```python
from build123d import *

# Parameters (mm, degrees)
F0_W         = 38.1
F0_H         = 38.1
F1_DEPTH     = 869.95
F2_W         = 12.7
F2_H         = 114.3
F2_H_2       = 25.4
F3_DEPTH     = 14.2875
F4_W         = 12.7
F4_H         = 114.3
F4_H_2       = 25.4
F5_DEPTH     = 14.2875
F6_T1_DEPTH  = 30.1625
F6_T3_DEPTH  = 12.7
F6_T5_DEPTH  = 30.1625
F6_T7_DEPTH  = 12.7
F6_T13_DEPTH = 28.575
F6_T17_DEPTH = 28.575
F6_T24_DEPTH = 28.575
F6_T28_DEPTH = 28.575
F6_T35_DEPTH = 28.575
F6_T39_DEPTH = 28.575
F6_T46_DEPTH = 28.575
F6_T50_DEPTH = 28.575


# Not quite as in the source:
# - a fillet or chamfer that OpenCascade refuses, or shapes differently, is made with other operations: its cross-section is extruded or revolved along the edge and cut away or added


with BuildPart() as f1:
    # F0 (on Top) → F1 (new body)
    with BuildSketch(Plane.XY):
        Rectangle(F0_W, F0_H)
    extrude(amount=-F1_DEPTH)

    # F2 (on face) → F3 (cut)
    with BuildSketch(Plane.XZ.offset(19.05)):
        with Locations((0, -76.2)):
            Rectangle(F2_W, F2_H)
        with Locations((0, -609.6)):
            Rectangle(F2_W, F2_H_2)
    extrude(amount=-F3_DEPTH, mode=Mode.SUBTRACT)

    # F4 (on face) → F5 (cut)
    with BuildSketch(Plane.YZ.offset(19.05)):
        with Locations((0, -76.2)):
            Rectangle(F4_W, F4_H)
        with Locations((0, -609.6)):
            Rectangle(F4_W, F4_H_2)
    extrude(amount=-F5_DEPTH, mode=Mode.SUBTRACT)

    # F6: fillet of radius 6.35 on 16 edges, made by hand

    # F6_s2 → F6_t1 (join)
    with BuildSketch(Plane.XZ.offset(-11.1125)):
        with BuildLine():
            ThreePointArc((-6.35, -25.4), (-4.4901280605, -20.9098719395), (0, -19.05))
            Line((0, -19.05), (-6.35, -19.05))
            Line((-6.35, -19.05), (-6.35, -25.4))
        make_face()
        with BuildLine():
            ThreePointArc((-6.35, -127), (-4.4901280605, -131.4901280605), (0, -133.35))
            Line((0, -133.35), (-6.35, -133.35))
            Line((-6.35, -133.35), (-6.35, -127))
        make_face()
        with BuildLine():
            ThreePointArc((-6.35, -603.25), (-4.4901280605, -598.7598719395), (0, -596.9))
            Line((0, -596.9), (-6.35, -596.9))
            Line((-6.35, -596.9), (-6.35, -603.25))
        make_face()
        with BuildLine():
            ThreePointArc((-6.35, -615.95), (-4.4901280605, -620.4401280605), (0, -622.3))
            Line((0, -622.3), (-6.35, -622.3))
            Line((-6.35, -622.3), (-6.35, -615.95))
        make_face()
    extrude(amount=F6_T1_DEPTH)

    # F6_s4 → F6_t3 (join)
    with BuildSketch(Plane.XZ.offset(6.35)):
        with BuildLine():
            ThreePointArc((6.35, -25.4), (4.4901280605, -20.9098719395), (0, -19.05))
            Line((0, -19.05), (6.35, -19.05))
            Line((6.35, -19.05), (6.35, -25.4))
        make_face()
        with BuildLine():
            ThreePointArc((0, -133.35), (4.4901280605, -131.4901280605), (6.35, -127))
            Line((6.35, -127), (6.35, -133.35))
            Line((6.35, -133.35), (0, -133.35))
        make_face()
        with BuildLine():
            ThreePointArc((6.35, -603.25), (4.4901280605, -598.7598719395), (0, -596.9))
            Line((0, -596.9), (6.35, -596.9))
            Line((6.35, -596.9), (6.35, -603.25))
        make_face()
        with BuildLine():
            ThreePointArc((0, -622.3), (4.4901280605, -620.4401280605), (6.35, -615.95))
            Line((6.35, -615.95), (6.35, -622.3))
            Line((6.35, -622.3), (0, -622.3))
        make_face()
    extrude(amount=F6_T3_DEPTH)

    # F6_s6 → F6_t5 (join)
    with BuildSketch(Plane.YZ.offset(-11.1125)):
        with BuildLine():
            ThreePointArc((0, -133.35), (4.4901280605, -131.4901280605), (6.35, -127))
            Line((6.35, -127), (6.35, -133.35))
            Line((6.35, -133.35), (0, -133.35))
        make_face()
        with BuildLine():
            ThreePointArc((0, -19.05), (4.4901280605, -20.9098719395), (6.35, -25.4))
            Line((6.35, -25.4), (6.35, -19.05))
            Line((6.35, -19.05), (0, -19.05))
        make_face()
        with BuildLine():
            ThreePointArc((0, -596.9), (4.4901280605, -598.7598719395), (6.35, -603.25))
            Line((6.35, -603.25), (6.35, -596.9))
            Line((6.35, -596.9), (0, -596.9))
        make_face()
        with BuildLine():
            ThreePointArc((0, -622.3), (4.4901280605, -620.4401280605), (6.35, -615.95))
            Line((6.35, -615.95), (6.35, -622.3))
            Line((6.35, -622.3), (0, -622.3))
        make_face()
    extrude(amount=F6_T5_DEPTH)

    # F6_s8 → F6_t7 (join)
    with BuildSketch(Plane.YZ.offset(6.35)):
        with BuildLine():
            ThreePointArc((0, -133.35), (-4.4901280605, -131.4901280605), (-6.35, -127))
            Line((-6.35, -127), (-6.35, -133.35))
            Line((-6.35, -133.35), (0, -133.35))
        make_face()
        with BuildLine():
            ThreePointArc((0, -19.05), (-4.4901280605, -20.9098719395), (-6.35, -25.4))
            Line((-6.35, -25.4), (-6.35, -19.05))
            Line((-6.35, -19.05), (0, -19.05))
        make_face()
        with BuildLine():
            ThreePointArc((0, -596.9), (-4.4901280605, -598.7598719395), (-6.35, -603.25))
            Line((-6.35, -603.25), (-6.35, -596.9))
            Line((-6.35, -596.9), (0, -596.9))
        make_face()
        with BuildLine():
            ThreePointArc((0, -622.3), (-4.4901280605, -620.4401280605), (-6.35, -615.95))
            Line((-6.35, -615.95), (-6.35, -622.3))
            Line((-6.35, -622.3), (0, -622.3))
        make_face()
    extrude(amount=F6_T7_DEPTH)


with BuildPart() as f6_tool11:
    # F6_s12 → F6_t13 (new body)
    with BuildSketch(Plane.XZ.offset(19.05)):
        with BuildLine():
            ThreePointArc((6.35, -25.4), (4.4901280605, -20.9098719395), (0, -19.05))
            Line((0, -19.05), (6.35, -19.05))
            Line((6.35, -19.05), (6.35, -25.4))
        make_face()
    extrude(amount=-F6_T13_DEPTH)

    split(bisect_by=Plane.XZ.offset(6.35), keep=Keep.BOTTOM)


with BuildPart() as f6_tool15:
    # F6_s16 → F6_t17 (new body)
    with BuildSketch(Plane.YZ.offset(19.05)):
        with BuildLine():
            ThreePointArc((0, -19.05), (-4.4901280605, -20.9098719395), (-6.35, -25.4))
            Line((-6.35, -25.4), (-6.35, -19.05))
            Line((-6.35, -19.05), (0, -19.05))
        make_face()
    extrude(amount=-F6_T17_DEPTH)

    split(bisect_by=Plane.YZ.offset(6.35), keep=Keep.BOTTOM)


with BuildPart() as f6_tool11_1:
    add(f6_tool11.part)

    # F6_t19: intersect F6_tool15
    add(f6_tool15.part, mode=Mode.INTERSECT)


with BuildPart() as f1_1:
    add(f1.part)

    # F6_t9: union F6_tool11
    add(f6_tool11_1.part)


with BuildPart() as f6_tool22:
    # F6_s23 → F6_t24 (new body)
    with BuildSketch(Plane.YZ.offset(19.05)):
        with BuildLine():
            ThreePointArc((0, -133.35), (-4.4901280605, -131.4901280605), (-6.35, -127))
            Line((-6.35, -127), (-6.35, -133.35))
            Line((-6.35, -133.35), (0, -133.35))
        make_face()
    extrude(amount=-F6_T24_DEPTH)

    split(bisect_by=Plane.YZ.offset(6.35), keep=Keep.BOTTOM)


with BuildPart() as f6_tool26:
    # F6_s27 → F6_t28 (new body)
    with BuildSketch(Plane.XZ.offset(19.05)):
        with BuildLine():
            ThreePointArc((0, -133.35), (4.4901280605, -131.4901280605), (6.35, -127))
            Line((6.35, -127), (6.35, -133.35))
            Line((6.35, -133.35), (0, -133.35))
        make_face()
    extrude(amount=-F6_T28_DEPTH)

    split(bisect_by=Plane.XZ.offset(6.35), keep=Keep.BOTTOM)


with BuildPart() as f6_tool22_1:
    add(f6_tool22.part)

    # F6_t30: intersect F6_tool26
    add(f6_tool26.part, mode=Mode.INTERSECT)


with BuildPart() as f1_2:
    add(f1_1.part)

    # F6_t20: union F6_tool22
    add(f6_tool22_1.part)


with BuildPart() as f6_tool33:
    # F6_s34 → F6_t35 (new body)
    with BuildSketch(Plane.XZ.offset(19.05)):
        with BuildLine():
            ThreePointArc((6.35, -603.25), (4.4901280605, -598.7598719395), (0, -596.9))
            Line((0, -596.9), (6.35, -596.9))
            Line((6.35, -596.9), (6.35, -603.25))
        make_face()
    extrude(amount=-F6_T35_DEPTH)

    split(bisect_by=Plane.XZ.offset(6.35), keep=Keep.BOTTOM)


with BuildPart() as f6_tool37:
    # F6_s38 → F6_t39 (new body)
    with BuildSketch(Plane.YZ.offset(19.05)):
        with BuildLine():
            ThreePointArc((0, -596.9), (-4.4901280605, -598.7598719395), (-6.35, -603.25))
            Line((-6.35, -603.25), (-6.35, -596.9))
            Line((-6.35, -596.9), (0, -596.9))
        make_face()
    extrude(amount=-F6_T39_DEPTH)

    split(bisect_by=Plane.YZ.offset(6.35), keep=Keep.BOTTOM)


with BuildPart() as f6_tool33_1:
    add(f6_tool33.part)

    # F6_t41: intersect F6_tool37
    add(f6_tool37.part, mode=Mode.INTERSECT)


with BuildPart() as f1_3:
    add(f1_2.part)

    # F6_t31: union F6_tool33
    add(f6_tool33_1.part)


with BuildPart() as f6_tool44:
    # F6_s45 → F6_t46 (new body)
    with BuildSketch(Plane.YZ.offset(19.05)):
        with BuildLine():
            ThreePointArc((0, -622.3), (-4.4901280605, -620.4401280605), (-6.35, -615.95))
            Line((-6.35, -615.95), (-6.35, -622.3))
            Line((-6.35, -622.3), (0, -622.3))
        make_face()
    extrude(amount=-F6_T46_DEPTH)

    split(bisect_by=Plane.YZ.offset(6.35), keep=Keep.BOTTOM)


with BuildPart() as f6_tool48:
    # F6_s49 → F6_t50 (new body)
    with BuildSketch(Plane.XZ.offset(19.05)):
        with BuildLine():
            ThreePointArc((0, -622.3), (4.4901280605, -620.4401280605), (6.35, -615.95))
            Line((6.35, -615.95), (6.35, -622.3))
            Line((6.35, -622.3), (0, -622.3))
        make_face()
    extrude(amount=-F6_T50_DEPTH)

    split(bisect_by=Plane.XZ.offset(6.35), keep=Keep.BOTTOM)


with BuildPart() as f6_tool44_1:
    add(f6_tool44.part)

    # F6_t52: intersect F6_tool48
    add(f6_tool48.part, mode=Mode.INTERSECT)


with BuildPart() as f1_4:
    add(f1_3.part)

    # F6_t42: union F6_tool44
    add(f6_tool44_1.part)


solid = f1_4.part
```
Geometry: final body of the model. Coordinates: model frame, mm. A direction names the side the tool comes from. Give positions to 0.01 mm unless a question says otherwise; leave off trailing zeros. Order: outer loops, then holes, each group sorted by start corner. A loop starts at its lowest first (then second) coordinate and runs counter-clockwise, first axis right, second up. Notation, with made-up numbers: (-30, 9) -> (-23, 9) arc R19 cw to (-23, 35) -> close; hole circle Ø4 at (66, 86). An arc over 180 degrees is marked (long way). Write each question's results on one line, items separated by ' | '. Start each with the question number.
1) Draft query along Z for faces 3 (the flat face through (0, 0, 0)), 4 (the flat face through (12, 6.35, -77)), 5 (the flat face through (-19.05, 0, -429)). Return one class per face: pulls with the +Z half, pulls with the -Z half, needs draft (parallel to the pull), parting line crosses it, or undercut.
2) Section A-A (y = -13). Return loops of the section in (x, z).
3) Line query: line 1 (Z direction, x = 9, y = 1); line 2 (Y direction, x = 14, z = -39); line 3 (Z direction, x = 4, y = -9). Output: solid intervals per line, ascending. Write a range as from..to.
4) Set-up query: faces 1 (the flat face through (0, 19.05, -429)), 2 (the flat face through (-6.35, -12, -77)). Return all of +Z, -Z, +X, -X, +Y, -Y with unobstructed straight access to the full face (end or side cutting, diameter ignored); none if empty.
5) Section B-B (z = -56.5). Return loops of the section in (x, y).
6) First-contact query: pin 1 (3.5 mm diameter, centred on y = -0.5, z = -60, fed in from +X); pin 2 (3.5 mm diameter, centred on x = -3.5, z = -62, fed in from -Y). Flat tips, straight axial feed; report the tip coordinate or a pass-through.
Calculated:
1) face 3: pulls with the +Z half | face 4: undercut | face 5: needs draft
2) outline: (-19.05, -869.95) -> (19.05, -869.95) -> (19.05, 0) -> (-19.05, 0) -> close; hole (-6.35, -615.95) arc R6.35 ccw to (6.35, -615.95) -> (6.35, -603.25) arc R6.35 ccw to (-6.35, -603.25) -> close; hole (-6.35, -127) arc R6.35 ccw to (6.35, -127) -> (6.35, -25.4) arc R6.35 ccw to (-6.35, -25.4) -> close
3) line 1: -869.95..-622.22, -596.98..-133.27, -19.13..0 | line 2: -19.05..-6.35, 6.35..19.05 | line 3: -869.95..-620.88, -598.32..-131.93, -20.47..0
4) face 1: +Z, -Z, +X, -X, +Y | face 2: -Y
5) outline: (-19.05, -19.05) -> (-6.35, -19.05) -> (-6.35, -4.76) -> (4.76, -4.76) -> (4.76, 6.35) -> (19.05, 6.35) -> (19.05, 19.05) -> (-19.05, 19.05) -> close; (6.35, -19.05) -> (19.05, -19.05) -> (19.05, -6.35) -> (6.35, -6.35) -> close
6) pin 1: x = 4.76 | pin 2: y = -4.76
